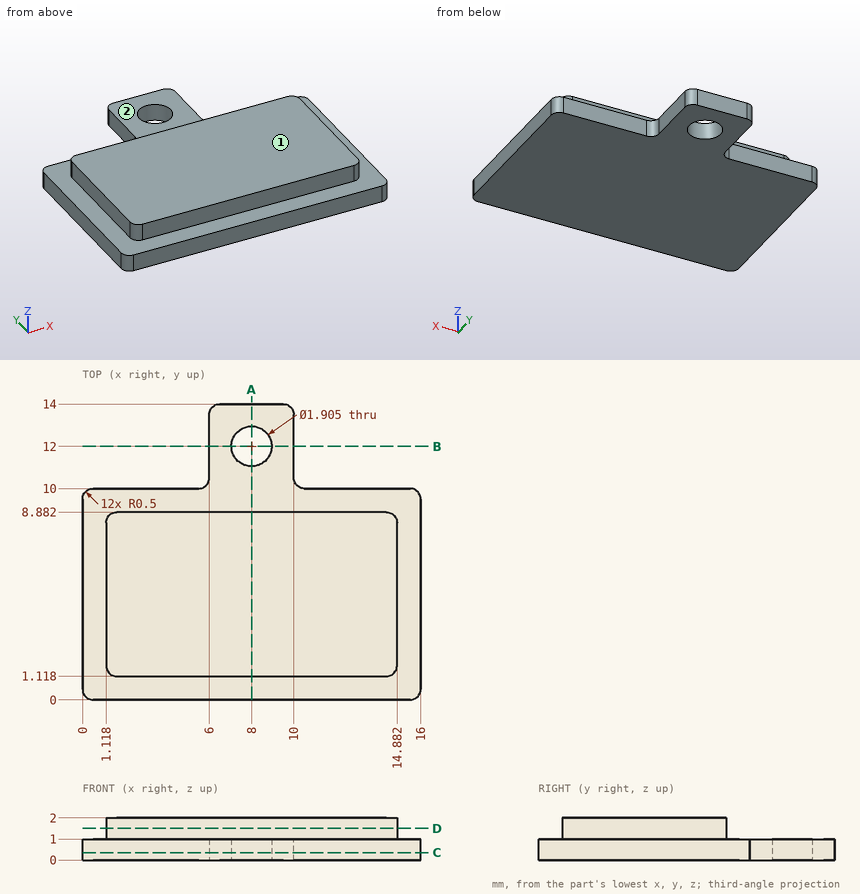
Verification items for this drawing (mm, ordinates from the low corner). A direction names the side the tool comes from. Coordinates: 2 decimals unless noted, no trailing zeros. Loops run counter-clockwise (first coordinate to the right, second up) from the corner with the lowest first, then second, coordinate; pieces in that order, holes last. Notation, with made-up numbers: (-6.5, -39.5) - (16.5, -39.5) arc R22 cw to (16.5, -12.5) - close; hole circle Ø11 at (1, 21). An arc over 180 degrees is marked (long way). Answer as a JSON object with one key per item and string values.
(1) Cross-section at C-C, the plane z = 0.35. Record the boundary of the cut face in (x, y) (1 decimal).
Response:
{"outline": "(0, 0.5) arc R0.5 ccw to (0.5, 0) - (15.5, 0) arc R0.5 ccw to (16, 0.5) - (16, 9.5) arc R0.5 ccw to (15.5, 10) - (10.5, 10) arc R0.5 cw to (10, 10.5) - (10, 13.5) arc R0.5 ccw to (9.5, 14) - (6.5, 14) arc R0.5 ccw to (6, 13.5) - (6, 10.5) arc R0.5 cw to (5.5, 10) - (0.5, 10) arc R0.5 ccw to (0, 9.5) - close; hole circle Ø1.9 at (8, 12)"}
(2) Access from +Z, -Z, +X, -X, +Y, -Y to the whole of each face (thin tool, end or side, straight path). Record for the marked faces 1 and 2.
Response:
{"face 1": "+Z, +X, -X, +Y, -Y", "face 2": "+Z"}
(3) Go/stop test with flat-tipped pins: pin 1 Ø1.1 at (x, z) = (2.5, 0.5) entering from +Y; pin 2 Ø0.5 at (y, z) = (4.5, 1.5) entering from +X; pin 3 Ø0.8 at (y, z) = (12.5, 0.5) entering from -X; pin 4 Ø1.5 at (x, y) = (3.5, 11.5) entering from -Z. Record where each tip stops, or that it passes through.
Response:
{"pin 1": "stops at y = 10", "pin 2": "stops at x = 14.88", "pin 3": "stops at x = 6", "pin 4": "passes through"}
(4) Scan lines: line 1 along X through (y, z) = (12, 0.5); line 2 along Y through (x, z) = (8, 0.75); line 3 along Y through (x, z) = (6.5, 1.2). Record each from-to range of solid material in increasing order.
Response:
{"line 1": "x = 6 to 7.05, 8.95 to 10", "line 2": "y = 0 to 11.05, 12.95 to 14", "line 3": "y = 1.12 to 8.88"}
(5) Cross-section at D-D, the plane z = 1.5. Record the boundary of the cut face in (x, y), then the cut area to 3 significant figures.
Response:
{"outline": "(1.12, 1.62) arc R0.5 ccw to (1.62, 1.12) - (14.38, 1.12) arc R0.5 ccw to (14.88, 1.62) - (14.88, 8.38) arc R0.5 ccw to (14.38, 8.88) - (1.62, 8.88) arc R0.5 ccw to (1.12, 8.38) - close", "area": "107 mm²"}
(6) Cross-section at A-A, the plane x = 8. Record the boundary of the cut face in (y, z).
Response:
{"outline": "(0, 0) - (11.05, 0) - (11.05, 1) - (8.88, 1) - (8.88, 2) - (1.12, 2) - (1.12, 1) - (0, 1) - close; (12.95, 0) - (14, 0) - (14, 1) - (12.95, 1) - close"}
(7) Cross-section at B-B, the plane y = 12. Record the boundary of the cut face in (x, z).
Response:
{"outline": "(6, 0) - (7.05, 0) - (7.05, 1) - (6, 1) - close; (8.95, 0) - (10, 0) - (10, 1) - (8.95, 1) - close"}
